Autodesk Inventor part; units mm, degrees
ref_plane "YZ Plane" through (0, 0, 0) normal (1, 0, 0) x (0, 1, 0)
ref_plane "XZ Plane" through (0, 0, 0) normal (0, 1, 0) x (-1, 0, 0)
ref_plane "XY Plane" through (0, 0, 0) normal (0, 0, 1) x (1, 0, 0)
sketch "Sketch1" plane through (0, 0, 0) normal (0, 1, 0) x (-1, 0, 0)
  circle A0 centre (0, 0) radius 203.2
  dimension "d0" = 406.4
extrude "Extrusion1" add sketch "Sketch1" along normal blind 9.525
sketch "Sketch2" plane through (0, 9.525, 0) normal (0, 1, 0) x (1, 0, 0)
  line L0 (0, 0) -> (64.6578, 64.6578) construction
  line L1 (0, 0) -> (91.44, 0) construction
  line L2 (64.6578, 64.6578) -> (102.0528, 86.2478)
  line L3 (64.6578, 64.6578) -> (107.8378, 64.6578) construction
  line L4 (64.6578, 64.6578) -> (64.6578, 107.8378)
  line L5 (64.6578, 64.6578) -> (27.2629, 86.2478)
  line L6 (64.6578, 64.6578) -> (27.2629, 43.0678)
  line L7 (64.6578, 64.6578) -> (64.6578, 21.4778)
  line L8 (64.6578, 64.6578) -> (102.0528, 43.0678)
  dimension "d3" = 91.44
  dimension "d4" = 45
  dimension "d5" = 43.18
  dimension "d6" = 30
  dimension "d9" = 360
hole "Hole1" at (64.6578, 9.525, -107.8378) at (27.2629, 9.525, -86.2478) at (27.2629, 9.525, -43.0678) at (102.0528, 9.525, -43.0678) at (102.0528, 9.525, -86.2478) at (64.6578, 9.525, -21.4778) direction (0, -1, 0) diameter 4.1402 end up to surface
sketch "Sketch3" plane through (0, 9.525, 0) normal (0, 1, 0) x (1, 0, 0)
  line L0 (0, 0) -> (64.6578, 64.6578) construction
  line L1 (0, 0) -> (91.44, 0) construction
  circle A0 centre (64.6578, 64.6578) radius 38.1
  dimension "d18" = 91.44
  dimension "d19" = 45
  dimension "d20" = 76.2
extrude "Extrusion2" cut sketch "Sketch3" against normal up to surface (9.525 mm away)
properties part number "2K8 stage" material "Copper"
Could you check a few things on this model? Use its own coordinates, in mm. Give positions to 0.01 mm unless a question says otherwise; leave off trailing zeros. Loops run counter-clockwise (first coordinate to the right, second up) from the corner with the lowest first, then second, coordinate; pieces in that order, holes last. Notation, with made-up numbers: (-6.5, -9.75) -> (10.5, -9.75) arc R8 ccw to (10.5, -2.75) -> close; hole circle Ø9 at (52.5, 37). An arc over 180 degrees is marked (long way). Put each result on its own line as item: value.
(1) Imagine slicing it at D-D on z = -136. Write out the boundary of the cut face in (x, y) (3 decimals).
Computed:
outline: (-150.978, 0) -> (150.978, 0) -> (150.978, 9.525) -> (-150.978, 9.525) -> close
(2) Please list where these lines run through material, in increasing order: probe 1 along X at (y, z) = (1, -67.5); probe 2 along Z at (x, y) = (49, 8); probe 3 along Z at (x, y) = (36, 4.5). Write a range as [from, to].
Computed:
probe 1: [-191.66, 26.66], [102.65, 191.66]
probe 2: [-197.2, -99.39], [-29.92, 197.2]
probe 3: [-199.99, -89.76], [-39.55, 199.99]
(3) I'm going to push flat-ended pins straight in: pin 1 Ø1 at (y, z) = (8, 59.5) entering from -X; pin 2 Ø4 at (y, z) = (6, 160.5) entering from +X; pin 3 Ø3.5 at (x, z) = (64.66, -21.48) entering from -Y; pin 4 Ø5 at (y, z) = (5, 62) entering from -X. Where does each tip first touch, or does it pass through?
Computed:
pin 1: x = -194.45
pin 2: x = 127.15
pin 3: through
pin 4: x = -194.29
(4) Imagine slicing it at C-C on z = 47. Write out the boundary of the cut face in (x, y) (3 decimals), plus the area to 3 significant figures.
Computed:
outline: (-197.69, 0) -> (197.69, 0) -> (197.69, 9.525) -> (-197.69, 9.525) -> close
area: 3,770 mm^2
(5) Imagine slicing it at A-A on z = -94. Write out the boundary of the cut face in (x, y) (3 decimals).
Computed:
outline: (-180.151, 0) -> (40.355, 0) -> (40.355, 9.525) -> (-180.151, 9.525) -> close; (88.961, 0) -> (180.151, 0) -> (180.151, 9.525) -> (88.961, 9.525) -> close
(6) Thinking about a two-plate mould opening in X: for faces 1 (the face through (44.05, 4.696, 198.368)), 2 (the face through (3, 0, 3)), 3 (the face through (101, 4.8, -76.1)), which applies, pulls with the +X half, pulls with the -X half, needs draft (parallel to the pull), parting line crosses it, or undercut?
Computed:
face 1: parting line crosses it
face 2: needs draft
face 3: undercut
(7) Imagine slicing it at B-B on y = 3.5. Write out the boundary of the cut face in (x, z).
Computed:
outline: circle Ø406.4 at (0, 0); hole circle Ø4.14 at (27.26, -86.25); hole circle Ø4.14 at (27.26, -43.07); hole circle Ø76.2 at (64.66, -64.66); hole circle Ø4.14 at (64.66, -107.84); hole circle Ø4.14 at (64.66, -21.48); hole circle Ø4.14 at (102.05, -86.25); hole circle Ø4.14 at (102.05, -43.07)
